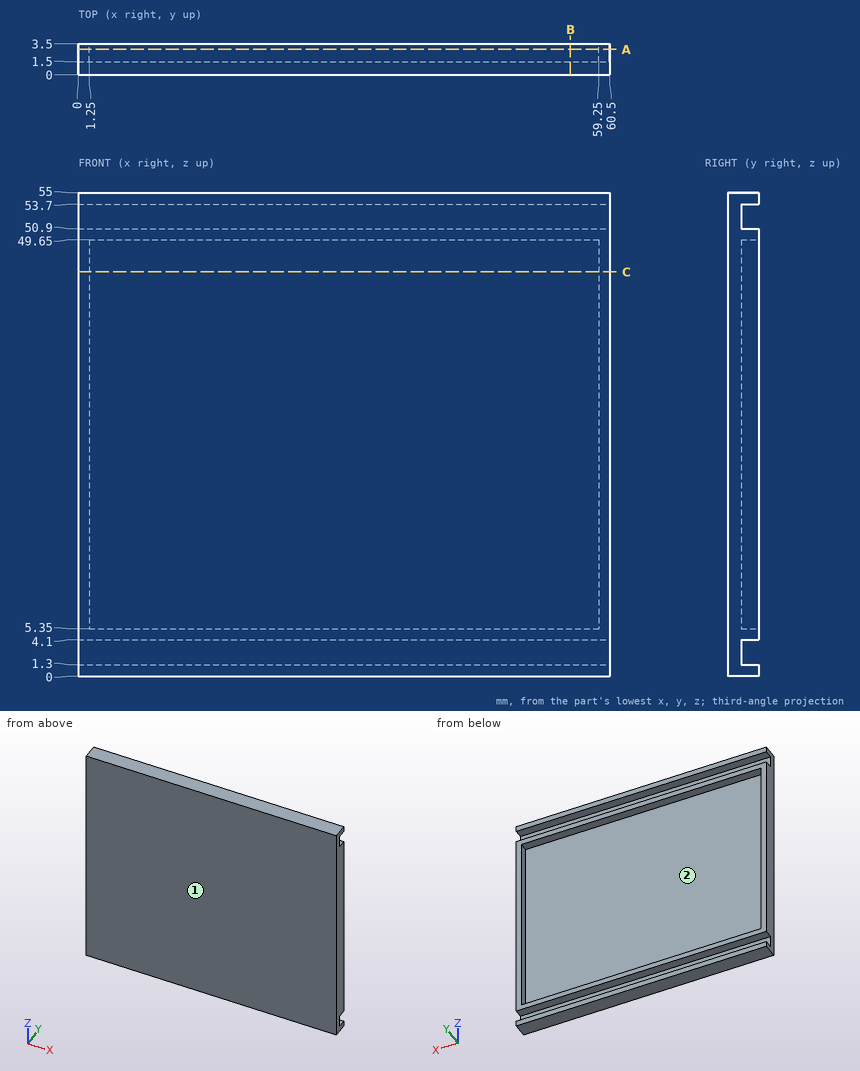
Geometry: see drawing. Coordinates: mm, zero at the bounding-box minimum. Give positions to 0.01 mm unless a question says otherwise; leave off trailing zeros. Loops run counter-clockwise (first coordinate to the right, second up) from the corner with the lowest first, then second, coordinate; pieces in that order, holes last. Notation, with made-up numbers: (-39, 74) -> (3, 74) arc R24 ccw to (3, 100) -> close; hole circle Ø2 at (80.5, -31). An arc over 180 degrees is marked (long way). Use one line per item in the form item = value.
Item 1: Section query B-B on x = 56. Output: boundary loops of the cut face in (y, z), and give its area (3 significant figures).
A:
outline = (0, 0) -> (3.5, 0) -> (3.5, 1.3) -> (1.5, 1.3) -> (1.5, 4.1) -> (3.5, 4.1) -> (3.5, 5.35) -> (1.5, 5.35) -> (1.5, 49.65) -> (3.5, 49.65) -> (3.5, 50.9) -> (1.5, 50.9) -> (1.5, 53.7) -> (3.5, 53.7) -> (3.5, 55) -> (0, 55) -> close
area = 92.7 mm^2
Item 2: Section query C-C on z = 46. Output: boundary loops of the cut face in (x, y), and give its area (4 significant figures).
A:
outline = (0, 0) -> (60.5, 0) -> (60.5, 3.5) -> (59.25, 3.5) -> (59.25, 1.5) -> (1.25, 1.5) -> (1.25, 3.5) -> (0, 3.5) -> close
area = 95.75 mm^2
Item 3: Line query: probe 1 along Z at (x, y) = (26, 1.75); probe 2 along X at (y, z) = (2.35, 24); probe 3 along Y at (x, z) = (10, 17). Output: solid intervals per line, ascending.
A:
probe_1 = 0 to 1.3, 4.1 to 5.35, 49.65 to 50.9, 53.7 to 55
probe_2 = 0 to 1.25, 59.25 to 60.5
probe_3 = 0 to 1.5
Item 4: Pin query (flat end, axial travel): P1, Ø13.5, axis at x = 29, z = 38, coming from the +Y side. Return the tip coordinate at first contact, or that it passes through.
A:
P1 = 1.5
Item 5: Section query A-A on y = 2.9. Output: boundary loops of the cut face in (x, z), and give its area (3 significant figures).
A:
outline = (0, 0) -> (60.5, 0) -> (60.5, 1.3) -> (0, 1.3) -> close; (0, 4.1) -> (60.5, 4.1) -> (60.5, 50.9) -> (0, 50.9) -> close; (0, 53.7) -> (60.5, 53.7) -> (60.5, 55) -> (0, 55) -> close; hole (1.25, 5.35) -> (59.25, 5.35) -> (59.25, 49.65) -> (1.25, 49.65) -> close
area = 419 mm^2
Item 6: Draft query along Z for the marked faces 1 and 2. Return one class per face: pulls with the +Z half, pulls with the -Z half, needs draft (parallel to the pull), parting line crosses it, or undercut.
A:
face_1 = needs draft
face_2 = undercut
